Geometry: final body of the model. Coordinates: model frame, mm. A direction names the side the tool comes from. Give positions to 0.01 mm unless a question says otherwise; leave off trailing zeros. Write each loop counter-clockwise with the first axis right and the second up, starting at its lowest first coordinate (ties: lowest second). Pieces come first, ordered by that corner, then holes. Notation, with made-up numbers: (32, 44) -> (63, 44) arc R24 cw to (63, 72) -> close; hole circle Ø1 at (14, 50.25). An arc over 180 degrees is marked (long way). Answer as a JSON object with one key per item and string values.
from build123d import *

# Parameters (mm, degrees)
F1_DEPTH = 1270
F2_R     = 1.5875
F3_DEPTH = 1270
F4_R     = 1.778
F5_DEPTH = 1270


with BuildPart() as f1:
    # F0 (on Right) → F1 (new body, symmetric)
    with BuildSketch(Plane.YZ):
        with BuildLine():
            Line((1.4224, 45.974), (0, 45.974))
            Line((0, 45.974), (0, 2.54))
            ThreePointArc((0, 2.54), (0.743949, 0.743949), (2.54, 0))
            Line((2.54, 0), (41.656, 0))
            Line((41.656, 0), (41.656, 1.4224))
            Line((41.656, 1.4224), (2.54, 1.4224))
            ThreePointArc((2.54, 1.4224), (1.749737, 1.749737), (1.4224, 2.54))
            Line((1.4224, 2.54), (1.4224, 45.974))
        make_face()
    extrude(amount=F1_DEPTH, both=True)

    # F2 (on Front) → F3 (intersect, symmetric)
    with BuildSketch(Plane.XZ):
        with BuildLine():
            ThreePointArc((19.939, 26.035), (0, 45.974), (-19.939, 26.035))
            Line((-19.939, 26.035), (-19.939, 0))
            Line((-19.939, 0), (19.939, 0))
            Line((19.939, 0), (19.939, 26.035))
        make_face()
        with Locations((-7.747, 11.727802)):
            Circle(F2_R, mode=Mode.SUBTRACT)
        with Locations((7.747, 11.727802)):
            Circle(F2_R, mode=Mode.SUBTRACT)
        with Locations((-15.494, 25.146)):
            Circle(F2_R, mode=Mode.SUBTRACT)
        with Locations((-7.747, 38.564198)):
            Circle(F2_R, mode=Mode.SUBTRACT)
        with BuildLine():
            Line((-6.477, 18.161), (-6.477, 32.131))
            ThreePointArc((-6.477, 32.131), (0, 38.608), (6.477, 32.131))
            Line((6.477, 32.131), (6.477, 18.161))
            ThreePointArc((6.477, 18.161), (0, 11.684), (-6.477, 18.161))
        make_face(mode=Mode.SUBTRACT)
        with Locations((15.494, 25.146)):
            Circle(F2_R, mode=Mode.SUBTRACT)
        with Locations((7.747, 38.564198)):
            Circle(F2_R, mode=Mode.SUBTRACT)
    extrude(amount=F3_DEPTH, both=True, mode=Mode.INTERSECT)

    # F4 (on Top) → F5 (intersect, symmetric)
    with BuildSketch(Plane.XY):
        with BuildLine():
            Line((-19.939, 38.481), (-19.939, 0))
            Line((-19.939, 0), (19.939, 0))
            Line((19.939, 0), (19.939, 38.481))
            ThreePointArc((19.939, 38.481), (19.009064, 40.726064), (16.764, 41.656))
            Line((16.764, 41.656), (-16.764, 41.656))
            ThreePointArc((-16.764, 41.656), (-19.009064, 40.726064), (-19.939, 38.481))
        make_face()
        with Locations((-14.9225, 10.16)):
            Circle(F4_R, mode=Mode.SUBTRACT)
        with Locations((14.9225, 10.16)):
            Circle(F4_R, mode=Mode.SUBTRACT)
        with Locations((-14.9225, 34.036)):
            Circle(F4_R, mode=Mode.SUBTRACT)
        with Locations((14.9225, 34.036)):
            Circle(F4_R, mode=Mode.SUBTRACT)
    extrude(amount=F5_DEPTH, both=True, mode=Mode.INTERSECT)


solid = f1.part
Q1. Material intervals for L1, parallel to X at y = 10.16, z = 0.8; L2, parallel to Z at x = -6.5, y = 12.5, sorted ascending. Write a range as from..to.
Values:
{"L1": "-19.94..-16.7, -13.14..13.14, 16.7..19.94", "L2": "0..1.42"}
Q2. Cut plane D-D (x = -8.5). Return the cut outline in (y, z).
Values:
{"outline": "(0, 2.54) arc R2.54 ccw to (2.54, 0) -> (41.66, 0) -> (41.66, 1.42) -> (2.54, 1.42) arc R1.12 cw to (1.42, 2.54) -> (1.42, 10.33) -> (0, 10.33) -> close; (0, 13.13) -> (1.42, 13.13) -> (1.42, 37.17) -> (0, 37.17) -> close; (0, 39.96) -> (1.42, 39.96) -> (1.42, 44.07) -> (0, 44.07) -> close"}
Q3. Cut plane B-B (x = 0). Return the cut outline in (y, z), and give its area (3 significant figures).
Values:
{"outline": "(0, 2.54) arc R2.54 ccw to (2.54, 0) -> (41.66, 0) -> (41.66, 1.42) -> (2.54, 1.42) arc R1.12 cw to (1.42, 2.54) -> (1.42, 11.68) -> (0, 11.68) -> close; (0, 38.61) -> (1.42, 38.61) -> (1.42, 45.97) -> (0, 45.97) -> close", "area": "83.2 mm²"}
Q4. Set-up query: faces 5 (the cylindrical face through (0.142, 0.701, 11.686)), 6 (the flat face through (9, 1.422, 19)), 7 (the cylindrical face through (-18.984, 40.751, 0.721)). Return all of +Z, -Z, +X, -X, +Y, -Y with unobstructed straight access to the full face (end or side cutting, diameter ignored); none if empty.
Values:
{"face 5": "+Y, -Y", "face 6": "+Z, +X, -X, +Y", "face 7": "+Z, -Z, -X, +Y"}
Q5. Mould query, pull axis Z, two halves, no side actions, for faces 1 (the cylindrical face through (19.034, 40.701, 0.721)), 2 (the cylindrical face through (-14.76, 0.72, 23.74)), 3 (the cylindrical face through (0.3, 1.8, 1.7)), 4 (the cylindrical face through (-7.01, 0.72, 10.32)). Classes: pulls with the +Z half, pulls with the -Z half, needs draft (parallel to the pull), parting line crosses it, or undercut.
Values:
{"face 1": "needs draft", "face 2": "undercut", "face 3": "pulls with the +Z half", "face 4": "undercut"}
Q6. Cut plane A-A (y = 10.16). Return the cut outline in (x, z).
Values:
{"outline": "(-19.94, 0) -> (-16.7, 0) -> (-16.7, 1.42) -> (-19.94, 1.42) -> close; (-13.14, 0) -> (13.14, 0) -> (13.14, 1.42) -> (-13.14, 1.42) -> close; (16.7, 0) -> (19.94, 0) -> (19.94, 1.42) -> (16.7, 1.42) -> close"}
Q7. Cut plane C-C (z = 34). Return the cut outline in (x, y).
Values:
{"outline": "(-18.28, 0) -> (-6.2, 0) -> (-6.2, 1.42) -> (-18.28, 1.42) -> close; (6.2, 0) -> (18.28, 0) -> (18.28, 1.42) -> (6.2, 1.42) -> close"}
Q8. First-contact query: P1, Ø4, axis at x = -15.494, z = 25.146, coming from the +Y side; P2, Ø4.5, axis at x = 14.92, y = 34.04, coming from the +Z side; P3, Ø1.6, axis at y = 1, z = 27.5, coming from the -X side. Flat tips, straight axial feed; report the tip coordinate or a pass-through.
Values:
{"P1": "y = 1.42", "P2": "z = 1.42", "P3": "x = -19.93"}
